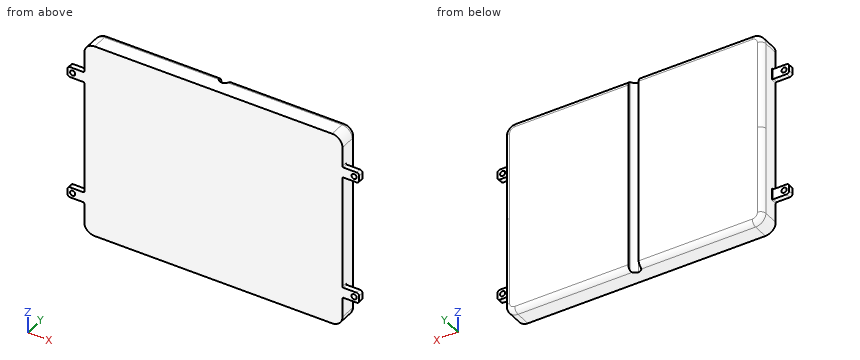
from build123d import *

# Parameters (mm, degrees)
BOSS_EXTRUDE1_DEPTH  = 10.16
SKETCH3_R            = 1.27
CUT_EXTRUDE1_DEPTH   = 10.16
SKETCH4_W            = 8.255
SKETCH4_H            = 7.62
CUT_EXTRUDE2_DEPTH   = 10.16
CUT_EXTRUDE3_DEPTH   = 69.596
FILLET1_R            = 2.54
FILLET2_R            = 0.508
FILLET3_R            = 1.27
FILLET1_OF_MIRROR3_R = 2.54
FILLET2_OF_MIRROR3_R = 0.508
FILLET3_OF_MIRROR3_R = 1.27


# Read off the part's stored shape, not the designer's step: Mirror4
with BuildPart() as part:
    # Sketch1 → Boss-Extrude1 (new body)
    with BuildSketch(Plane(origin=(0, 0, 0), x_dir=(1, 0, 0), z_dir=(0, 1, 0))):
        with BuildLine():
            Line((-58.188733064, -33.517116066), (5.311266936, -33.517116066))
            Line((5.311266936, -33.517116066), (5.311266936, 14.742883934))
            Line((5.311266936, 14.742883934), (-53.108733064, 14.742883934))
            ThreePointArc((-53.108733064, 14.742883934), (-56.700835512, 13.254986382), (-58.188733064, 9.662883934))
            Line((-58.188733064, 9.662883934), (-58.188733064, -0.370116066))
            Line((-58.188733064, -0.370116066), (-66.443733064, -0.370116066))
            Line((-66.443733064, -0.370116066), (-66.443733064, -5.450116066))
            Line((-66.443733064, -5.450116066), (-58.188733064, -5.450116066))
            Line((-58.188733064, -5.450116066), (-58.188733064, -33.517116066))
        make_face()
    boss_extrude1 = extrude(amount=BOSS_EXTRUDE1_DEPTH)

    # Sketch3 → Cut-Extrude1 (cut)
    with BuildSketch(Plane(origin=(0, 10.16, 0), x_dir=(1, 0, 0), z_dir=(0, 1, 0))):
        with Locations(Location((-63.903733064, -2.910116066, 0), (0, 0, 270))):
            Circle(SKETCH3_R)
    cut_extrude1 = extrude(amount=-CUT_EXTRUDE1_DEPTH, mode=Mode.SUBTRACT)

    # Sketch4 → Cut-Extrude2 (cut)
    with BuildSketch(Plane.XY.offset(5.450116066)):
        with Locations((-62.316233064, 6.35)):
            Rectangle(SKETCH4_W, SKETCH4_H)
    cut_extrude2 = extrude(amount=-CUT_EXTRUDE2_DEPTH, mode=Mode.SUBTRACT)

    # Sketch5 → Cut-Extrude3 (cut)
    with BuildSketch(Plane.XY.offset(33.517116066)):
        with BuildLine():
            Line((5.311266936, 10.16), (5.311266936, 8.89))
            Line((5.311266936, 8.89), (5.311266936, 6.35))
            ThreePointArc((5.311266936, 6.35), (3.515215712, 7.093948776), (2.771266936, 8.89))
            Line((2.771266936, 8.89), (2.771266936, 10.16))
            Line((2.771266936, 10.16), (5.311266936, 10.16))
        make_face()
    cut_extrude3 = extrude(amount=-CUT_EXTRUDE3_DEPTH, mode=Mode.SUBTRACT)

    # Fillet1
    fillet1_edges = [part.edges().sort_by_distance(p)[0] for p in [
        (-25.168733064, 10.16, -14.742883934),
        (-56.700835512, 10.16, -13.254986382),
        (-58.188733064, 10.16, 11.927116066),
    ]]
    fillet(fillet1_edges, radius=FILLET1_R)

    # Fillet2
    fillet2_edges = [part.edges().sort_by_distance(p)[0] for p in [
        (-58.188733064, 1.27, 5.450116066),
        (-58.188733064, 1.27, 0.370116066),
        (-58.188733064, 2.54, 2.910116066),
    ]]
    fillet(fillet2_edges, radius=FILLET2_R)

    # Fillet3
    fillet3_edges = [part.edges().sort_by_distance(p)[0] for p in [
        (-66.443733064, 1.27, 5.450116066),
        (-66.443733064, 1.27, 0.370116066),
    ]]
    fillet(fillet3_edges, radius=FILLET3_R)

    # Mirror3: Boss-Extrude1, Cut-Extrude1, Cut-Extrude2, Cut-Extrude3 across plane
    add(boss_extrude1.mirror(Plane(origin=(-58.188733064, 10.16, 33.517116066), x_dir=(1, 0, 0), z_dir=(0, 0, -1))))
    add(cut_extrude1.mirror(Plane(origin=(-58.188733064, 10.16, 33.517116066), x_dir=(1, 0, 0), z_dir=(0, 0, -1))), mode=Mode.SUBTRACT)
    add(cut_extrude2.mirror(Plane(origin=(-58.188733064, 10.16, 33.517116066), x_dir=(1, 0, 0), z_dir=(0, 0, -1))), mode=Mode.SUBTRACT)
    add(cut_extrude3.mirror(Plane(origin=(-58.188733064, 10.16, 33.517116066), x_dir=(1, 0, 0), z_dir=(0, 0, -1))), mode=Mode.SUBTRACT)

    # Fillet1 of Mirror3
    fillet1_of_mirror3_edges = [part.edges().sort_by_distance(p)[0] for p in [
        (-25.168733064, 10.16, 81.777116066),
        (-56.700835512, 10.16, 80.289218515),
        (-58.188733064, 10.16, 55.107116066),
    ]]
    fillet(fillet1_of_mirror3_edges, radius=FILLET1_OF_MIRROR3_R)

    # Fillet2 of Mirror3
    fillet2_of_mirror3_edges = [part.edges().sort_by_distance(p)[0] for p in [
        (-58.188733064, 1.27, 61.584116066),
        (-58.188733064, 1.27, 66.664116066),
        (-58.188733064, 2.54, 64.124116066),
    ]]
    fillet(fillet2_of_mirror3_edges, radius=FILLET2_OF_MIRROR3_R)

    # Fillet3 of Mirror3
    fillet3_of_mirror3_edges = [part.edges().sort_by_distance(p)[0] for p in [
        (-66.443733064, 1.27, 61.584116066),
        (-66.443733064, 1.27, 66.664116066),
    ]]
    fillet(fillet3_of_mirror3_edges, radius=FILLET3_OF_MIRROR3_R)

    # Mirror4: part across plane


with BuildPart() as part_1:
    add(part.part)
    add(part.part.mirror(Plane(origin=(5.311266936, 10.16, -14.742883934), x_dir=(0, 0, 1), z_dir=(-1, 0, 0))))


solid = part_1.part
Source: CAD feature listing. Evaluate the final solid. Frame: model axes, mm. Coordinates: 2 decimals unless noted, no trailing zeros. Write each loop counter-clockwise with the first axis right and the second up, starting at its lowest first coordinate (ties: lowest second). Pieces come first, ordered by that corner, then holes. Notation, with made-up numbers: M 31.5,39.5 L 66.5,39.5 A26 cw 66.5,59.5 Z; hole C 29,-34 d5. An arc over 180 degrees is marked long. Use a Markdown table: item, result.
1) Section A-A, the plane z = 22.5. Output: boundary loops of the cut face in (x, y), then the cut area to 3 significant figures.
Conclusion:
| item | result |
|---|---|
| outline | M -58.19,0 L 68.81,0 L 68.81,7.62 A2.54 ccw 66.27,10.16 L 7.85,10.16 L 7.85,8.89 A2.54 cw 2.77,8.89 L 2.77,10.16 L -55.65,10.16 A2.54 ccw -58.19,7.62 Z |
| area | 1,270 mm^2 |
2) Ray query, L1, parallel to X at y = 1.5, z = 67; L2, parallel to X at y = 9.25, z = 65. Return the intervals inside material, ascending.
Conclusion:
| item | result |
|---|---|
| L1 | x = -58.22 to 68.84 |
| L2 | x = -57.6 to 2.77, 7.85 to 68.22 |
3) First-contact query: pin 1 Ø1.4 at (y, z) = (9.5, 46) entering from +X; pin 2 Ø1 at (y, z) = (7, 4.5) entering from +X; pin 3 Ø0.8 at (x, y) = (72, 1) entering from +Z. Flat tips, straight axial feed; report the tip coordinate or a pass-through.
Conclusion:
| item | result |
|---|---|
| pin 1 | stops at x = 68.52 |
| pin 2 | stops at x = 68.81 |
| pin 3 | stops at z = 66.66 |
